Build history of the part. All positions in model axes, mm. A direction names the side the tool comes from. Give positions to 0.01 mm unless a question says otherwise; leave off trailing zeros. Order: outer loops, then holes, each group sorted by start corner. A loop starts at its lowest first (then second) coordinate and runs counter-clockwise, first axis right, second up. Notation, with made-up numbers: (62.5, -3.75) -> (112.5, -3.75) arc R19 cw to (112.5, 28.25) -> close; hole circle Ø6 at (-30, -7). An arc over 180 degrees is marked (long way). One line per item, written item: value. Start each with the question number.
(1) Saw through at A-A on y = 26. Give the cut face in (x, z), plus the area to 3 significant figures.
(2) Saw through at C-C on z = -29.5. Give the cut face in (x, y).
(3) Probe line 1 (X direction, y = 47, z = -22.5); line 2 (X direction, y = 5.75, z = -15); line 3 (Y direction, x = 33.5, z = -17). List the from-to ranges inside material, lowest first.
(4) Two-plate mould, pull along Z, no slides. Class faces 4 (the cylindrical face through (78.1, 4.93, -15.15)), 5 (the flat face through (62, 9, 0)), 6 (the flat face through (-15, 45, -17)): +Z half, -Z half, draft (parallel to the pull), parting line (faces both ways), or undercut.
(5) Pin check, flat tips, straight feed: pin 1 (3 mm diameter, centred on y = 68.5, z = -25.5, fed in from +X); pin 2 (2 mm diameter, centred on x = 107.5, z = -25.5, fed in from -Y); pin 3 (1.5 mm diameter, centred on x = 50, z = -22.5, fed in from +Y). Stop position of each tip, or through.
(6) Saw through at B-B on x = 35.5. Give the cut face in (y, z), plus the area to 3 significant figures.
(7) Which spindle directions (+Z, -Z, +X, -X, +Y, -Y) get a long thin tool onto all of the face, cutting with end or side? Do faces 1 (the flat face through (115, 45, -17)), 2 (the cylindrical face through (26.757, 4.93, -13.736)), 3 (the flat face through (102.1, 25.5, -17.3)). Say none if no direction does.
(8) Saw through at D-D on z = -15. Give the cut face in (x, y), plus the area to 3 significant figures.
```python
from build123d import *

# Parameters (mm, degrees)
SKETCH1_W                = 100
SKETCH1_H                = 35
BOSS_EXTRUDE1_DEPTH      = 10
BOSS_EXTRUDE2_DEPTH      = 35
SKETCH3_R                = 17.5
BOSS_EXTRUDE3_DEPTH      = 130
CHAMFER1_SIZE            = 15
CUT_EXTRUDE1_DEPTH       = 158.896326746
M6_CLEARANCE_HOLE1_D     = 6.6
M6_CLEARANCE_HOLE1_DEPTH = 10


with BuildPart() as part:
    # Sketch1 → Boss-Extrude1 (new body)
    with BuildSketch(Plane(origin=(0, 0, 0), x_dir=(1, 0, 0), z_dir=(0, 1, 0))):
        with Locations((50, 17.5)):
            Rectangle(SKETCH1_W, SKETCH1_H)
    extrude(amount=BOSS_EXTRUDE1_DEPTH)

    # Sketch2 → Boss-Extrude2 (add)
    with BuildSketch(Plane.XY):
        Polygon((0, 0), (-30, 35), (-30, 65), (-15, 65), (-15, 40.548861143), (11.184738123, 10), align=None)
        Polygon((115, 40.548861143), (88.815261877, 10), (100, 0), (130, 35), (130, 65), (115, 65), align=None)
    extrude(amount=-BOSS_EXTRUDE2_DEPTH)

    # Sketch3 → Boss-Extrude3 (add)
    with BuildSketch(Plane.ZY.offset(-115)):
        with Locations(Location((-17.5, 65, 0), (0, 0, 180))):
            Circle(SKETCH3_R)
    extrude(amount=BOSS_EXTRUDE3_DEPTH)

    # Chamfer1
    # the kernel refuses this chamfer: 15 mm, written as the material it adds along each edge
    with BuildSketch(Plane(origin=(-15, 65, 38.575244819), x_dir=(-0.9996219169112968, -0.02749587661058678, 0), z_dir=(0, 0, -1))) as chamfer1_piece_1_section:
        Polygon((CHAMFER1_SIZE * 0.999621916911, CHAMFER1_SIZE * 0.0274958766106), (-CHAMFER1_SIZE * 0.0274958766106, CHAMFER1_SIZE * 0.999621916911), (0, 0), align=None)
    chamfer1_piece_1 = extrude(amount=112.150489639, mode=Mode.PRIVATE)
    chamfer1_piece_1 = chamfer1_piece_1 & Plane(origin=(-20.149822061, 65, -17.5), x_dir=(0, 0, -1), z_dir=(1, 0, 0)) * Cylinder(17.5, 285, mode=Mode.PRIVATE)
    add(chamfer1_piece_1)
    with BuildSketch(Plane(origin=(115, 65, 38.575244819), x_dir=(0.9996219169112966, -0.02749587661058679, 0), z_dir=(0, 0, -1))) as chamfer1_piece_2_section:
        Polygon((CHAMFER1_SIZE * 0.999621916911, -CHAMFER1_SIZE * 0.0274958766106), (-CHAMFER1_SIZE * 0.0274958766106, -CHAMFER1_SIZE * 0.999621916911), (0, 0), align=None)
    chamfer1_piece_2 = extrude(amount=112.150489639, mode=Mode.PRIVATE)
    chamfer1_piece_2 = chamfer1_piece_2 & Plane(origin=(120.149822061, 65, -17.5), x_dir=(0, 0, -1), z_dir=(1, 0, 0)) * Cylinder(17.5, 285, mode=Mode.PRIVATE)
    add(chamfer1_piece_2)

    # Sketch4 → Cut-Extrude1 (cut, through all)
    with BuildSketch(Plane(origin=(0, 0, -35), x_dir=(-1, 0, 0), z_dir=(0, 0, -1))):
        Polygon((-130, 65), (-112.5, 82.5), (-130, 82.5), align=None)
        Polygon((12.5, 82.5), (30, 82.5), (30, 65), align=None)
    extrude(amount=-CUT_EXTRUDE1_DEPTH, mode=Mode.SUBTRACT)

    # M6 Clearance Hole1
    with Locations(Plane(origin=(0, 10, 0), x_dir=(1, 0, 0), z_dir=(0, 1, 0))):
        with Locations((29.805261877, 15), (74.805261877, 15)):
            Hole(M6_CLEARANCE_HOLE1_D / 2, depth=M6_CLEARANCE_HOLE1_DEPTH)


solid = part.part
```
Results below:
1. outline: (-22.29, -35) -> (-2.53, -35) -> (-2.53, 0) -> (-22.29, 0) -> close; (102.53, -35) -> (122.29, -35) -> (122.29, 0) -> (102.53, 0) -> close
1. area: 1,380 mm²
2. outline: (-30, 35) -> (0, 0) -> (100, 0) -> (130, 35) -> (130, 65) -> (117.26, 77.74) -> (-17.26, 77.74) -> (-30, 65) -> close; hole (-15, 40.55) -> (11.18, 10) -> (88.82, 10) -> (115, 40.55) -> (115, 52.26) -> (-15, 52.26) -> close
3. line 1: x = -30 to -15, 115 to 130
3. line 2: x = -4.93 to 26.51, 33.11 to 71.51, 78.11 to 104.93
3. line 3: y = 0 to 10, 47.51 to 82.49
4. face 4: undercut
4. face 5: +Z half
4. face 6: draft
5. pin 1: stops at x = 128
5. pin 2: stops at y = 7.58
5. pin 3: stops at y = 81.98
6. outline: (0, -35) -> (10, -35) -> (10, 0) -> (0, 0) -> close; circle Ø35 at (65, -17.5)
6. area: 1,310 mm²
7. face 1: none
7. face 2: -Y
7. face 3: +Z, -Z
8. outline: (-30, 35) -> (0, 0) -> (26.51, 0) -> (26.51, 10) -> (11.18, 10) -> (-15, 40.55) -> (-15, 47.68) -> (115, 47.68) -> (115, 40.55) -> (88.82, 10) -> (78.11, 10) -> (78.11, 0) -> (100, 0) -> (130, 35) -> (130, 65) -> (112.68, 82.32) -> (-12.68, 82.32) -> (-30, 65) -> close; (33.11, 0) -> (71.51, 0) -> (71.51, 10) -> (33.11, 10) -> close
8. area: 7,590 mm²
